from build123d import *

# Parameters (mm, degrees)
F1_DEPTH = 17.526
F2_DEPTH = 1.27
F3_R     = 5.715
F4_DEPTH = 17.526
F6_R     = 1.1811
F7_DEPTH = 20.828


with BuildPart() as f1:
    # F0 (on Top) → F1 (new body)
    with BuildSketch(Plane.XY):
        with BuildLine():
            ThreePointArc((2.032, -6.016101), (5.158764, -3.702654), (6.35, 0))
            ThreePointArc((6.35, 0), (-3.702654, 5.158764), (-2.032, -6.016101))
            ThreePointArc((-2.032, -6.016101), (0, -6.35), (2.032, -6.016101))
        make_face()
        with BuildLine():
            ThreePointArc((2.032, -6.016101), (0, -6.35), (-2.032, -6.016101))
            Line((-2.032, -6.016101), (-2.032, -13.97))
            ThreePointArc((-2.032, -13.97), (0, -16.002), (2.032, -13.97))
            Line((2.032, -13.97), (2.032, -6.016101))
        make_face()
    extrude(amount=F1_DEPTH)

    # F0 (on Top) → F2 (join)
    with BuildSketch(Plane.XY):
        with BuildLine():
            ThreePointArc((2.032, -6.016101), (0, -6.35), (-2.032, -6.016101))
            Line((-2.032, -6.016101), (-2.032, -13.97))
            ThreePointArc((-2.032, -13.97), (0, -16.002), (2.032, -13.97))
            Line((2.032, -13.97), (2.032, -6.016101))
        make_face()
    extrude(amount=-F2_DEPTH)

    # F3 (on face) → F4 (cut, through all)
    with BuildSketch(Plane.XY.offset(17.526)):
        Circle(F3_R)
    extrude(amount=-F4_DEPTH, mode=Mode.SUBTRACT)

    # F6 (on offset) → F7 (cut)
    with BuildSketch(Plane.XZ.offset(-6.35)):
        with Locations((0, 2.413)):
            Circle(F6_R)
        with Locations((0, 5.461)):
            Circle(F6_R)
        with Locations((0, 8.509)):
            Circle(F6_R)
        with Locations((0, 11.557)):
            Circle(F6_R)
        with Locations((0, 14.605)):
            Circle(F6_R)
    extrude(amount=F7_DEPTH, mode=Mode.SUBTRACT)


solid = f1.part
Can you work these out from the model? Positions are in its coordinate system, mm. A direction names the side the tool comes from. Round coordinates to 2 decimals unless told otherwise and drop trailing zeros. Write each loop counter-clockwise with the first axis right and the second up, starting at its lowest first coordinate (ties: lowest second). Pieces come first, ordered by that corner, then holes. Notation, with made-up numbers: M 46,16.25 L 102,16.25 A25 cw 102,40.25 Z; hole C 25,28.25 d11. An arc over 180 degrees is marked long. Use a Markdown table: item, result.
Item 1: I want a section at A-A (x = -2.5). List the corners of the cut face in (y, z) for me, and give its area (3 significant figures).
Found:
| item | result |
|---|---|
| outline | M -5.84,0 L -5.14,0 L -5.14,17.53 L -5.84,17.53 Z; M 5.14,0 L 5.84,0 L 5.84,17.53 L 5.14,17.53 Z |
| area | 24.5 mm2 |
Item 2: We'd pull the mould along Y, two halves only. Please class faces 4 (the face through (0, -14.478, 9)), 5 (the face through (0, -11, -1.27)), 6 (the face through (2.64, -5.07, 8.89)): released by +Y, released by -Y, zero draft, split by the parting line, or undercut.
Found:
| item | result |
|---|---|
| face 4 | released by +Y |
| face 5 | zero draft |
| face 6 | undercut |
Item 3: For pin 1 Ø1.9 at (x, z) = (0.5, 5.5) entering from +Y; pin 2 Ø2 at (x, z) = (-4.5, 8) entering from +Y; pin 3 Ø1.2 at (x, z) = (0, 2) entering from +Y, each with a flat end and sliding along its axis, tell me the tip position at first contact or that it passes through.
Found:
| item | result |
|---|---|
| pin 1 | stops at y = 6.31 |
| pin 2 | stops at y = 5.3 |
| pin 3 | stops at y = -14.48 |
Item 4: If I drill on line 1 along Z through (x, y) = (0, -7.75); line 2 along Z through (x, y) = (0, 6.05); line 3 along X through (y, z) = (-6.5, 8.5), over which ranges is the centre line in solid material (lowest first)? Write a range as [from, to].
Found:
| item | result |
|---|---|
| line 1 | z = [-1.27, 1.23], [3.59, 4.28], [6.64, 7.33], [9.69, 10.38], [12.74, 13.42], [15.79, 17.53] |
| line 2 | z = [0, 1.23], [3.59, 4.28], [6.64, 7.33], [9.69, 10.38], [12.74, 13.42], [15.79, 17.53] |
| line 3 | x = [-2.03, -1.18], [1.18, 2.03] |
Item 5: I want a section at C-C (x = 0). State how many separate pieces and enclosed holes the cut face has, and give its area (3 significant figures).
Found:
| item | result |
|---|---|
| separate pieces | 7 |
| enclosed holes | 0 |
| area | 92.7 mm2 |
Item 6: Which directions (+Z, -Z, +X, -X, +Y, -Y) give clear straight access to the entire face, cutting with the end or side of a thin tool? Please do faces 1 (the face through (0.03, -6.35, -0.63)), 2 (the face through (2.032, -10, 8)), 3 (the face through (0.545, -9.97, 7.461)).
Found:
| item | result |
|---|---|
| face 1 | -Z, +Y |
| face 2 | +Z, -Z, +X, -Y |
| face 3 | +Y |
Item 7: I want a section at B-B (y = -3.25). List the corners of the cut face in (x, z) for me.
Found:
| item | result |
|---|---|
| outline | M -5.46,0 L -4.7,0 L -4.7,17.53 L -5.46,17.53 Z; M 4.7,0 L 5.46,0 L 5.46,17.53 L 4.7,17.53 Z |
Item 8: I want a section at D-D (y = -13.5). List the corners of the cut face in (x, z) for me (3 decimals), and give its area (3 significant figures).
Found:
| item | result |
|---|---|
| outline | M -2.032,-1.27 L 2.032,-1.27 L 2.032,17.526 L -2.032,17.526 Z; hole C 0,2.413 d2.362; hole C 0,5.461 d2.362; hole C 0,8.509 d2.362; hole C 0,11.557 d2.362; hole C 0,14.605 d2.362 |
| area | 54.5 mm2 |
